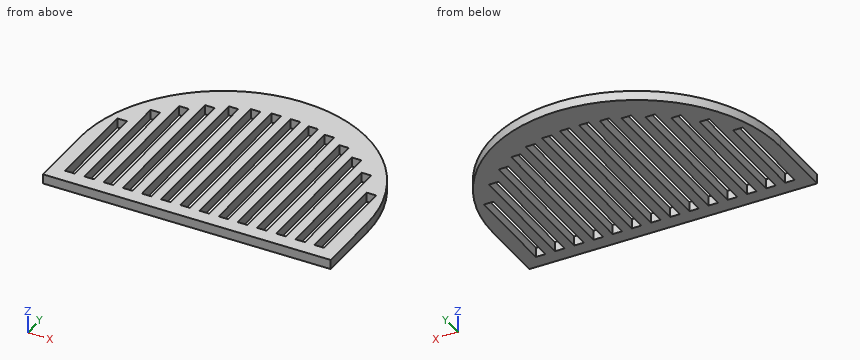
```python
from build123d import *

# Parameters (mm, degrees)
P_IDAT_VYSUNUT_M1_DEPTH  = 10
ODEBRAT_VYSUNUT_M1_REACH = 374.156
SKICA2_W                 = 10
SKICA2_H                 = 99.833147735
LINPOLE2_START           = 15
LINPOLE2_OUTLINE_W       = 10
LINPOLE2_OUTLINE_H       = 10
LINPOLE2_DEPTH           = 126.980390272
LINPOLE2_START_2         = 141.980390272
LINPOLE2_2_OUTLINE_W     = 10
LINPOLE2_2_OUTLINE_H     = 10
LINPOLE2_2_DEPTH         = 30.684601342
LINPOLE2_3_OUTLINE_W     = 10
LINPOLE2_3_OUTLINE_H     = 10
LINPOLE2_3_DEPTH         = 99.833147735
LINPOLE2_START_3         = 172.664991614
LINPOLE2_4_OUTLINE_W     = 10
LINPOLE2_4_OUTLINE_H     = 10
LINPOLE2_4_DEPTH         = 14.304392953
LINPOLE2_5_OUTLINE_W     = 10
LINPOLE2_5_OUTLINE_H     = 10
LINPOLE2_5_DEPTH         = 18.019609728
LINPOLE2_6_OUTLINE_W     = 10
LINPOLE2_6_OUTLINE_H     = 10
LINPOLE2_6_DEPTH         = 8.756364623
LINPOLE2_START_4         = 186.969384567
LINPOLE2_7_OUTLINE_W     = 10
LINPOLE2_7_OUTLINE_H     = 10
LINPOLE2_7_DEPTH         = 2.696910904


# Read off the part's stored shape, not the designer's step: LinPole2
with BuildPart() as part:
    # Skica1 → Přidat vysunutím1 (new body)
    with BuildSketch(Plane.XY):
        with BuildLine():
            Line((0, 0), (0, 70))
            ThreePointArc((0, 70), (150, 220), (300, 70))
            Line((300, 70), (300, 0))
            Line((300, 0), (0, 0))
        make_face()
    extrude(amount=P_IDAT_VYSUNUT_M1_DEPTH)

    # Skica2 → Odebrat vysunutím1 (cut, up to next)
    with BuildSketch(Plane(origin=(0, 0, 0), x_dir=(-1, 0, 0), z_dir=(0, 0, -1)), mode=Mode.PRIVATE) as odebrat_vysunut_m1_sk1:
        with Locations((-280, 64.916573868)):
            Rectangle(SKICA2_W, SKICA2_H)
    odebrat_vysunut_m1_tool1 = extrude(odebrat_vysunut_m1_sk1.sketch, amount=-ODEBRAT_VYSUNUT_M1_REACH, mode=Mode.PRIVATE) & part.part
    add(odebrat_vysunut_m1_tool1.solids().sort_by_distance((280, 64.916574, 0))[0], mode=Mode.SUBTRACT)

    # LinPole2 outline → LinPole2 (cut)
    with BuildSketch(Plane(origin=(0, 0, 0), x_dir=(1, 0, 0), z_dir=(0, 1, 0)).offset(LINPOLE2_START)):
        with Locations((40, -5)):
            Rectangle(LINPOLE2_OUTLINE_W, LINPOLE2_OUTLINE_H)
        with Locations((60, -5)):
            Rectangle(LINPOLE2_OUTLINE_W, LINPOLE2_OUTLINE_H)
        with Locations((80, -5)):
            Rectangle(LINPOLE2_OUTLINE_W, LINPOLE2_OUTLINE_H)
        with Locations((100, -5)):
            Rectangle(LINPOLE2_OUTLINE_W, LINPOLE2_OUTLINE_H)
        with Locations((120, -5)):
            Rectangle(LINPOLE2_OUTLINE_W, LINPOLE2_OUTLINE_H)
        with Locations((140, -5)):
            Rectangle(LINPOLE2_OUTLINE_W, LINPOLE2_OUTLINE_H)
        with Locations((160, -5)):
            Rectangle(LINPOLE2_OUTLINE_W, LINPOLE2_OUTLINE_H)
        with Locations((180, -5)):
            Rectangle(LINPOLE2_OUTLINE_W, LINPOLE2_OUTLINE_H)
        with Locations((200, -5)):
            Rectangle(LINPOLE2_OUTLINE_W, LINPOLE2_OUTLINE_H)
        with Locations((220, -5)):
            Rectangle(LINPOLE2_OUTLINE_W, LINPOLE2_OUTLINE_H)
        with Locations((240, -5)):
            Rectangle(LINPOLE2_OUTLINE_W, LINPOLE2_OUTLINE_H)
        with Locations((260, -5)):
            Rectangle(LINPOLE2_OUTLINE_W, LINPOLE2_OUTLINE_H)
    extrude(amount=LINPOLE2_DEPTH, mode=Mode.SUBTRACT)

    # LinPole2 2 outline → LinPole2 2 (cut)
    with BuildSketch(Plane(origin=(0, 0, 0), x_dir=(1, 0, 0), z_dir=(0, 1, 0)).offset(LINPOLE2_START_2)):
        with Locations((80, -5)):
            Rectangle(LINPOLE2_2_OUTLINE_W, LINPOLE2_2_OUTLINE_H)
        with Locations((100, -5)):
            Rectangle(LINPOLE2_2_OUTLINE_W, LINPOLE2_2_OUTLINE_H)
        with Locations((120, -5)):
            Rectangle(LINPOLE2_2_OUTLINE_W, LINPOLE2_2_OUTLINE_H)
        with Locations((140, -5)):
            Rectangle(LINPOLE2_2_OUTLINE_W, LINPOLE2_2_OUTLINE_H)
        with Locations((160, -5)):
            Rectangle(LINPOLE2_2_OUTLINE_W, LINPOLE2_2_OUTLINE_H)
        with Locations((180, -5)):
            Rectangle(LINPOLE2_2_OUTLINE_W, LINPOLE2_2_OUTLINE_H)
        with Locations((200, -5)):
            Rectangle(LINPOLE2_2_OUTLINE_W, LINPOLE2_2_OUTLINE_H)
        with Locations((220, -5)):
            Rectangle(LINPOLE2_2_OUTLINE_W, LINPOLE2_2_OUTLINE_H)
    extrude(amount=LINPOLE2_2_DEPTH, mode=Mode.SUBTRACT)

    # LinPole2 3 outline → LinPole2 3 (cut)
    with BuildSketch(Plane(origin=(0, 0, 0), x_dir=(1, 0, 0), z_dir=(0, 1, 0)).offset(LINPOLE2_START)):
        with Locations((20, -5)):
            Rectangle(LINPOLE2_3_OUTLINE_W, LINPOLE2_3_OUTLINE_H)
    extrude(amount=LINPOLE2_3_DEPTH, mode=Mode.SUBTRACT)

    # LinPole2 4 outline → LinPole2 4 (cut)
    with BuildSketch(Plane(origin=(0, 0, 0), x_dir=(1, 0, 0), z_dir=(0, 1, 0)).offset(LINPOLE2_START_3)):
        with Locations((120, -5)):
            Rectangle(LINPOLE2_4_OUTLINE_W, LINPOLE2_4_OUTLINE_H)
        with Locations((140, -5)):
            Rectangle(LINPOLE2_4_OUTLINE_W, LINPOLE2_4_OUTLINE_H)
        with Locations((160, -5)):
            Rectangle(LINPOLE2_4_OUTLINE_W, LINPOLE2_4_OUTLINE_H)
        with Locations((180, -5)):
            Rectangle(LINPOLE2_4_OUTLINE_W, LINPOLE2_4_OUTLINE_H)
    extrude(amount=LINPOLE2_4_DEPTH, mode=Mode.SUBTRACT)

    # LinPole2 5 outline → LinPole2 5 (cut)
    with BuildSketch(Plane(origin=(0, 0, 0), x_dir=(1, 0, 0), z_dir=(0, 1, 0)).offset(LINPOLE2_START_2)):
        with Locations((60, -5)):
            Rectangle(LINPOLE2_5_OUTLINE_W, LINPOLE2_5_OUTLINE_H)
        with Locations((240, -5)):
            Rectangle(LINPOLE2_5_OUTLINE_W, LINPOLE2_5_OUTLINE_H)
    extrude(amount=LINPOLE2_5_DEPTH, mode=Mode.SUBTRACT)

    # LinPole2 6 outline → LinPole2 6 (cut)
    with BuildSketch(Plane(origin=(0, 0, 0), x_dir=(1, 0, 0), z_dir=(0, 1, 0)).offset(LINPOLE2_START_3)):
        with Locations((100, -5)):
            Rectangle(LINPOLE2_6_OUTLINE_W, LINPOLE2_6_OUTLINE_H)
        with Locations((200, -5)):
            Rectangle(LINPOLE2_6_OUTLINE_W, LINPOLE2_6_OUTLINE_H)
    extrude(amount=LINPOLE2_6_DEPTH, mode=Mode.SUBTRACT)

    # LinPole2 7 outline → LinPole2 7 (cut)
    with BuildSketch(Plane(origin=(0, 0, 0), x_dir=(1, 0, 0), z_dir=(0, 1, 0)).offset(LINPOLE2_START_4)):
        with Locations((140, -5)):
            Rectangle(LINPOLE2_7_OUTLINE_W, LINPOLE2_7_OUTLINE_H)
        with Locations((160, -5)):
            Rectangle(LINPOLE2_7_OUTLINE_W, LINPOLE2_7_OUTLINE_H)
    extrude(amount=LINPOLE2_7_DEPTH, mode=Mode.SUBTRACT)


solid = part.part
```
Check sheet for the modelled part. Datum: model origin and axes. Units: mm. Coordinates: 2 decimals unless noted, no trailing zeros. Loops run counter-clockwise (first coordinate to the right, second up) from the corner with the lowest first, then second, coordinate; pieces in that order, holes last.
1) Material ranges on probe 1 along X at (y, z) = (189, 1.5); probe 2 along Y at (x, z) = (80, 5.5) (3 decimals); probe 3 along Y at (x, z) = (237, 8.5), recorded low to high.
2) Sectioned sample at B-B (z = 2.5). Count the separate pieces of the cut face and the enclosed holes in it, and give its area (3 significant figures).
3) Gauge pin test, flat ends, axial feed: pin 1 (3 mm diameter, centred on x = 92, z = 8.5, fed in from +Y); pin 2 (2 mm diameter, centred on x = 259, z = 6, fed in from +Y); pin 3 (3 mm diameter, centred on y = 82, z = 3, fed in from -X). Record the tip position at first contact, or that the pin passes through.
4) Sectioned sample at A-A (x = 41.5). Record the boundary of the cut face in (y, z), and give its area (3 significant figures).
Check sheet entries:
1. probe 1: x = 58.68 to 135, 145 to 155, 165 to 241.32
1. probe 2: y = 0 to 15, 172.665 to 202.665
1. probe 3: y = 0 to 15, 160 to 192.19
2. separate pieces: 1
2. enclosed holes: 14
2. area: 35,500 mm2
3. pin 1: stops at y = 208.95
3. pin 2: stops at y = 174.1
3. pin 3: stops at x = 0.37
4. outline: (0, 0) - (15, 0) - (15, 10) - (0, 10) - close; (141.98, 0) - (173.57, 0) - (173.57, 10) - (141.98, 10) - close
4. area: 466 mm2
